Input: part model. Units: mm. Frame: model coordinates. A direction names the side the tool comes from. Coordinates: 2 decimals unless noted, no trailing zeros. Loops run counter-clockwise (first coordinate to the right, second up) from the corner with the lowest first, then second, coordinate; pieces in that order, holes last. Notation, with made-up numbers: (9, 20.25) -> (48, 20.25) arc R18 cw to (48, 32.25) -> close; hole circle Ø8 at (44.25, -14.75). An arc over 180 degrees is marked (long way). Put each result on its own line as item: value. Start each with the question number.
1) Cut plane D-D (x = -21.5). Return the cut outline in (y, z), plus the area to 3 significant figures.
2) Contact query for flat-ended pins moving along their axis: P1, Ø8, axis at y = -54.5, z = 39.5, coming from the +X side; P2, Ø1, axis at x = 16.5, y = -6, coming from the -Z side; P3, Ø1, axis at x = -59, z = -13.5, coming from the -Y side; P4, Ø4, axis at y = -48, z = 39.5, coming from the -X side. Output: stop coordinate, or through.
3) Cut plane C-C (z = 27). Return the cut outline in (x, y).
4) Set-up query: faces 4 (the flat face through (-1, 5, -1)), 5 (the flat face through (-1, -5, -1)). Return all of +Z, -Z, +X, -X, +Y, -Y with unobstructed straight access to the full face (end or side cutting, diameter ignored); none if empty.
5) Cut plane A-A (x = -90). Return the cut outline in (y, z), plus the area to 3 significant figures.
6) Pull-direction query (Z, two-part tool) for faces 1 (the flat face through (-1, 0, 50)), 2 (the flat face through (-100, 0, 1)), 3 (the conical face through (-83.09, -40.49, -42.87)); classes: pulls with the +Z half, pulls with the -Z half, needs draft (parallel to the pull), parting line crosses it, or undercut.
7) Cut plane B-B (y = -39). Return the cut outline in (x, z).
8) Material intervals for L1, parallel to X at y = -55, z = -43 (3 decimals); L2, parallel to Y at x = 80, z = -20; L3, parallel to X at y = -25, z = -41.5, sorted ascending.
from build123d import *

# Parameters (mm, degrees)
SKETCH1_W           = 200
SKETCH1_H           = 100
BOSS_EXTRUDE1_DEPTH = 5
SKETCH2_R           = 8.75
SKETCH3_R           = 6.25
SKETCH2_4_R         = 8.75
SKETCH3_3_R         = 6.25
SKETCH2_5_R         = 8.75
SKETCH3_4_R         = 6.25
SKETCH2_6_R         = 8.75
SKETCH3_5_R         = 6.25


with BuildPart() as part:
    # Sketch1 → Boss-Extrude1 (new, symmetric)
    with BuildSketch(Plane(origin=(0, 0, 0), x_dir=(1, 0, 0), z_dir=(0, 1, 0))):
        Rectangle(SKETCH1_W, SKETCH1_H)
    extrude(amount=BOSS_EXTRUDE1_DEPTH, both=True)

    # Sketch2 → Loft1 section 0
    with BuildSketch(Plane.XZ.offset(5)):
        with Locations((-90, -40)):
            Circle(SKETCH2_R)
    # Sketch3 → Loft1 section 1
    with BuildSketch(Plane(origin=(0, -75, 0), x_dir=(1, 0, 0), z_dir=(0, 1, 0))):
        with Locations((-90, 40)):
            Circle(SKETCH3_R)
    loft()

    # Sketch2<4> → Loft2 section 0
    with BuildSketch(Plane.XZ.offset(5)):
        with Locations((-90, 40)):
            Circle(SKETCH2_4_R)
    # Sketch3<3> → Loft2 section 1
    with BuildSketch(Plane(origin=(0, -75, 0), x_dir=(1, 0, 0), z_dir=(0, 1, 0))):
        with Locations((-90, -40)):
            Circle(SKETCH3_3_R)
    loft()

    # Sketch2<5> → Loft3 section 0
    with BuildSketch(Plane.XZ.offset(5)):
        with Locations((90, 40)):
            Circle(SKETCH2_5_R)
    # Sketch3<4> → Loft3 section 1
    with BuildSketch(Plane(origin=(0, -75, 0), x_dir=(1, 0, 0), z_dir=(0, 1, 0))):
        with Locations((90, -40)):
            Circle(SKETCH3_4_R)
    loft()

    # Sketch2<6> → Loft4 section 0
    with BuildSketch(Plane.XZ.offset(5)):
        with Locations((90, -40)):
            Circle(SKETCH2_6_R)
    # Sketch3<5> → Loft4 section 1
    with BuildSketch(Plane(origin=(0, -75, 0), x_dir=(1, 0, 0), z_dir=(0, 1, 0))):
        with Locations((90, 40)):
            Circle(SKETCH3_5_R)
    loft()


solid = part.part
Results found:
1. outline: (-5, -50) -> (5, -50) -> (5, 50) -> (-5, 50) -> close
1. area: 1,000 mm2
2. P1: stops at x = 97.12
2. P2: passes through
2. P3: stops at y = -5
2. P4: stops at x = -97.28
3. outline: (-100, -5) -> (100, -5) -> (100, 5) -> (-100, 5) -> close
4. face 4: +Z, -Z, +X, -X, +Y
4. face 5: -Y
5. outline: (-75, -46.25) -> (-5, -48.75) -> (-5, -50) -> (5, -50) -> (5, 50) -> (-5, 50) -> (-5, 48.75) -> (-75, 46.25) -> (-75, 33.75) -> (-5, 31.25) -> (-5, -31.25) -> (-75, -33.75) -> close
5. area: 3,100 mm2
6. face 1: pulls with the +Z half
6. face 2: needs draft
6. face 3: undercut
7. outline: circle Ø15.07 at (-90, -40); circle Ø15.07 at (-90, 40); circle Ø15.07 at (90, -40); circle Ø15.07 at (90, 40)
8. L1: x = -96.285 to -83.715, 83.715 to 96.285
8. L2: y = -5 to 5
8. L3: x = -97.89 to -82.11, 82.11 to 97.89
